CAD build for the part. Positions are in the model's coordinates, mm. A direction names the side the tool comes from. Give positions to 0.01 mm unless a question says otherwise; leave off trailing zeros. Loops run counter-clockwise (first coordinate to the right, second up) from the corner with the lowest first, then second, coordinate; pieces in that order, holes last.
Item 1: Mould opens along Y. For faces 3 (the cylindrical face through (-151.894, -8.004, 8.381)), 4 (the cylindrical face through (71.65, 76.63, 8.38)), 5 (the flat face through (-12.542, 137.933, 8.381)), 6 (the flat face through (-122.75, -47.21, 8.38)) say: released by +Y, released by -Y, zero draft, split by the parting line, or undercut.
Item 2: Which spindle directions (+Z, -Z, +X, -X, +Y, -Y) get a long thin tool onto all of the face, cutting with end or side? Do faces 1 (the cylindrical face through (54.177, 138.744, 4.943)), 2 (the cylindrical face through (-132.634, -5.797, 8.381)). Say none if no direction does.
Item 3: Saw through at D-D on y = 11.1. Give the number of separate pieces and of enclosed holes in the cut face, plus the area to 3 significant figures.
Item 4: Drop flat-ended pins along their axis: P1, Ø1.5, axis at y = 49.5, z = 2.5, coming from the -X side; P2, Ø6.5, axis at x = 75.43, y = -75.43, coming from the +Z side; P3, Ø5, axis at y = 93.5, z = 2.5, coming from the +X side; P4, Ø3, axis at y = -25, z = 15, coming from the +X side. Give the stop position or say it passes through.
Item 5: Saw through at A-A on y = 115.44. Give the cut face in (x, z).
Item 6: Saw through at B-B on x = -52.65. Give the cut face in (y, z) (3 decimals).
Item 7: Saw through at C-C on x = 98.5. Give the cut face in (y, z).
Item 8: Probe probe 1 along Y at (x, z) = (50.73, 15.5); probe 2 along X at (y, z) = (-93.77, 15.25); probe 3 along X at (y, z) = (-3, 14.75). List the from-to ranges inside material, lowest first.
from build123d import *

# Parameters (mm, degrees)
SKETCH1_R                         = 37.475
SKETCH1_R_2                       = 4
SKETCH1_R_3                       = 6
SKETCH1_R_4                       = 1.687903887
BOSS_EXTRUDE1_DEPTH               = 17
M10X1_25_TAPPED_HOLE1_D           = 8.8
M10X1_25_TAPPED_HOLE1_ON_FACE_2_D = 8.8
F_6_0MM_DOWEL_HOLE1_D             = 6
F_3_8_16_TAPPED_HOLE1_D           = 7.9375
CHAMFER1_SIZE                     = 1
CBORE_FOR_M10_SHCS1_AT_2_COUNT    = 2
CBORE_FOR_M10_SHCS1_AT_2_PITCH    = 133.628097719
CBORE_FOR_M10_SHCS1_AT_3_COUNT    = 2
CBORE_FOR_M10_SHCS1_AT_3_PITCH    = 223.034803562
CBORE_FOR_M10_SHCS1_AT_4_COUNT    = 2
CBORE_FOR_M10_SHCS1_AT_4_PITCH    = 246.886744075


with BuildPart() as part:
    # Sketch1 → Boss-Extrude1 (new body)
    with BuildSketch(Plane.XY):
        with BuildLine():
            Line((-147.843963588, -16.38510421), (-96.939761408, -78.915668014))
            ThreePointArc((-96.939761408, -78.915668014), (71.436269945, -102.576114843), (107.636664229, 63.55586923))
            Line((107.636664229, 63.55586923), (63.646399708, 138.056704308))
            ThreePointArc((63.646399708, 138.056704308), (57.374372961, 143.878133995), (48.939902164, 145.322801944))
            Line((48.939902164, 145.322801944), (-75.770097836, 130.332801944))
            ThreePointArc((-75.770097836, 130.332801944), (-82.520736984, 127.771091264), (-87.292449774, 122.352212454))
            Line((-87.292449774, 122.352212454), (-150.342449774, 0.922212454))
            ThreePointArc((-150.342449774, 0.922212454), (-151.87610245, -8.133185025), (-147.843963588, -16.38510421))
        make_face()
        Circle(SKETCH1_R, mode=Mode.SUBTRACT)
        with Locations((-73.98, 115.44)):
            Circle(SKETCH1_R_2, mode=Mode.SUBTRACT)
        with Locations((50.73, 130.43)):
            Circle(SKETCH1_R_3, mode=Mode.SUBTRACT)
        with Locations((110.87, 11.1)):
            Circle(SKETCH1_R_3, mode=Mode.SUBTRACT)
        with Locations((107.78, -40.88)):
            Circle(SKETCH1_R_4, mode=Mode.SUBTRACT)
        with Locations((54.67, -92.57)):
            Circle(SKETCH1_R_3, mode=Mode.SUBTRACT)
        with Locations((-52.65, -93.77)):
            Circle(SKETCH1_R_3, mode=Mode.SUBTRACT)
        with Locations((-137.03, -5.99)):
            Circle(SKETCH1_R_2, mode=Mode.SUBTRACT)
    extrude(amount=BOSS_EXTRUDE1_DEPTH)

    # M10x1.25 Tapped Hole1 (through all)
    with Locations(Plane(origin=(-73.98, 115.44, 17), x_dir=(1, 0, 0), z_dir=(0, 0, 1))):
        with Locations((0, 0)):
            Hole(M10X1_25_TAPPED_HOLE1_D / 2)

    # M10x1.25 Tapped Hole1 on face 2 (through all)
    with Locations(Plane(origin=(-137.03, -5.99, 0), x_dir=(1, 0, 0), z_dir=(0, 0, 1))):
        with Locations((0, 0)):
            Hole(M10X1_25_TAPPED_HOLE1_ON_FACE_2_D / 2)

    # Ø6.0mm Dowel Hole1 (through all)
    with Locations(Plane(origin=(107.78, -40.88, 17), x_dir=(1, 0, 0), z_dir=(0, 0, 1))):
        with Locations((0, 0)):
            Hole(F_6_0MM_DOWEL_HOLE1_D / 2)

    # 3/8-16 Tapped Hole1 (through all)
    with Locations(Plane(origin=(-75.434151417, 75.434151417, 17), x_dir=(1, 0, 0), z_dir=(0, 0, 1))):
        with Locations((0, 0), (0, -150.868302834), (150.868302834, -150.868302834), (150.868302834, 0)):
            Hole(F_3_8_16_TAPPED_HOLE1_D / 2)

    # Chamfer1
    chamfer1_edges = [part.edges().sort_by_distance(p)[0] for p in [
        (-37.475, 0, 17),
    ]]
    chamfer(chamfer1_edges, length=CHAMFER1_SIZE)

    # Sketch12 → CBORE for M10 SHCS1 (revolve, cut)
    with BuildSketch(Plane(origin=(50.73, 130.43, 0), x_dir=(0, 1, 0), z_dir=(1, 0, 0))):
        Polygon((0, 0), (0, 17), (5.25, 17), (5.25, 10), (9, 10), (9, 0.025), (9.025, 0), align=None)
    cbore_for_m10_shcs1 = revolve(axis=Axis((50.73, 130.43, -6.35), (0, 0, 1)), mode=Mode.SUBTRACT)

    # CBORE for M10 SHCS1 at 2: CBORE for M10 SHCS1 ×2
    with Locations(*[Vector(0.45005504850082595, -0.8930008137280274, 0) * (i * CBORE_FOR_M10_SHCS1_AT_2_PITCH) for i in range(1, CBORE_FOR_M10_SHCS1_AT_2_COUNT)]):
        add(cbore_for_m10_shcs1, mode=Mode.SUBTRACT)

    # CBORE for M10 SHCS1 at 3: CBORE for M10 SHCS1 ×2
    with Locations(*[Vector(0.017665404399104877, -0.9998439545686197, 0) * (i * CBORE_FOR_M10_SHCS1_AT_3_PITCH) for i in range(1, CBORE_FOR_M10_SHCS1_AT_3_COUNT)]):
        add(cbore_for_m10_shcs1, mode=Mode.SUBTRACT)

    # CBORE for M10 SHCS1 at 4: CBORE for M10 SHCS1 ×2
    with Locations(*[Vector(-0.4187345107866802, -0.9081086991523866, 0) * (i * CBORE_FOR_M10_SHCS1_AT_4_PITCH) for i in range(1, CBORE_FOR_M10_SHCS1_AT_4_COUNT)]):
        add(cbore_for_m10_shcs1, mode=Mode.SUBTRACT)


solid = part.part
Results below:
1. face 3: split by the parting line
1. face 4: undercut
1. face 5: released by +Y
1. face 6: released by -Y
2. face 1: -Z
2. face 2: +Z, -Z
3. separate pieces: 3
3. enclosed holes: 0
3. area: 3,100 mm2
4. P1: stops at x = -125.51
4. P2: passes through
4. P3: stops at x = 91.43
4. P4: stops at x = 122.77
5. outline: (-90.88, 0) - (-78.38, 0) - (-78.38, 17) - (-90.88, 17) - close; (-69.58, 0) - (77, 0) - (77, 17) - (-69.58, 17) - close
6. outline: (-113.371, 0) - (-102.795, 0) - (-102.77, 0.025) - (-102.77, 10) - (-99.77, 10) - (-99.77, 17) - (-113.371, 17) - close; (-87.77, 10) - (-84.77, 10) - (-84.77, 0.025) - (-84.745, 0) - (133.112, 0) - (133.112, 17) - (-87.77, 17) - close
7. outline: (-76.96, 0) - (79.03, 0) - (79.03, 17) - (-76.96, 17) - close
8. probe 1: y = -114.24 to -97.1, -88.04 to 124.43, 136.43 to 145.43
8. probe 2: x = -82.66 to -58.65, -46.65 to 48.79, 60.55 to 82.66
8. probe 3: x = -151.73 to -140.26, -133.8 to -37.35, 37.35 to 124.96
